```python
from build123d import *

# Parameters (mm, degrees)
Y_KSEKLIK_EKSTR_ZYON1_DEPTH = 10
PAH1_SIZE                   = 3
RADYUS1_R                   = 3


with BuildPart() as part:
    # Çizim1 → Yükseklik-Ekstrüzyon1 (new body)
    with BuildSketch(Plane.XY):
        Polygon((0, 0), (0, 110), (90, 0), align=None)
    extrude(amount=Y_KSEKLIK_EKSTR_ZYON1_DEPTH)

    # Pah1
    pah1_edges = [part.edges().sort_by_distance(p)[0] for p in [
        (0, 0, 5),
    ]]
    chamfer(pah1_edges, length=PAH1_SIZE)

    # Radyus1
    radyus1_edges = [part.edges().sort_by_distance(p)[0] for p in [
        (0, 110, 5),
        (90, 0, 5),
    ]]
    fillet(radyus1_edges, radius=RADYUS1_R)


solid = part.part
```
For this review, take the finished solid that the model builds, in its own axes (mm). Coordinates: 2 decimals unless noted, no trailing zeros. Write each loop counter-clockwise with the first axis right and the second up, starting at its lowest first coordinate (ties: lowest second). Pieces come first, ordered by that corner, then holes. Notation, with made-up numbers: (77, -33) -> (100, -33) arc R19 ccw to (100, -18) -> close; hole circle Ø1 at (7.25, 16). An arc over 180 degrees is marked (long way). Put each result on its own line as item: value.
Q1. Take a section at B-B, the plane y = 33. State the section outline as (x, z) points.
From the geometry:
outline: (0, 0) -> (63, 0) -> (63, 10) -> (0, 10) -> close
Q2. Take a section at C-C, the plane x = 36. State the section outline as (y, z) points, then the cut area to 3 significant figures.
From the geometry:
outline: (0, 0) -> (66, 0) -> (66, 10) -> (0, 10) -> close
area: 660 mm2
Q3. Wall thickness on L1, parallel to Y at x = 12.5, z = 1.5; L2, parallel to Y at x = 42.5, z = 4; L3, parallel to X at y = 41.5, z = 4: over which ranges is each line inside the solid? List them lowest first.
From the geometry:
L1: y = 0 to 94.72
L2: y = 0 to 58.06
L3: x = 0 to 56.05
Q4. Take a section at A-A, the plane z = 5. State the section outline as (x, y) points, then the cut area to 3 significant figures.
From the geometry:
outline: (0, 3) -> (3, 0) -> (83.67, 0) arc R3 ccw to (85.99, 4.9) -> (5.32, 103.5) arc R3 ccw to (0, 101.6) -> close
area: 4,920 mm2
